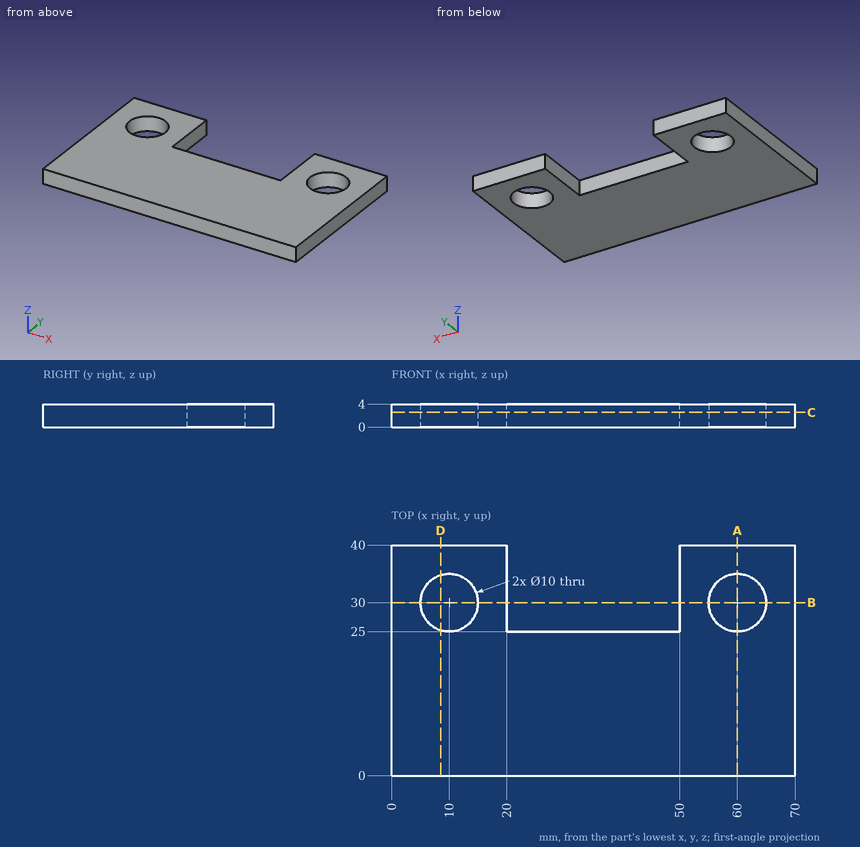
Verification items for this drawing (mm, ordinates from the low corner). Round coordinates to 2 decimals unless told otherwise and drop trailing zeros. Order: outer loops, then holes, each group sorted by start corner. A loop starts at its lowest first (then second) coordinate and runs counter-clockwise, first axis right, second up. Notation, with made-up numbers: M -37.75,31 L -7.75,31 A20 cw -7.75,43 Z; hole C 0.5,28 d11. An arc over 180 degrees is marked long. Answer in a Markdown table with one row per item. Add a question column.
Item 1: Depth check by flat-ended pin: pin 1 Ø1.2 at (x, z) = (31.5, 1.5) entering from +Y. Enter the tip coordinate at first touch or a pass-through.
Item 2: Sectioned sample at A-A, the plane x = 60. Enter the section's corners in (y, z), plus the area to 3 significant figures.
Item 3: Material ranges on L1, parallel to X at y = 30, z = 2.85; L2, parallel to Y at x = 10, z = 1.75; L3, parallel to X at y = 26.5, z = 2.8, recorded low to high. Write a range as [from, to].
Item 4: Sectioned sample at C-C, the plane z = 2.55. Enter the section's corners in (x, y).
Item 5: Sectioned sample at D-D, the plane x = 8.5. Enter the section's corners in (y, z), plus the area to 3 significant figures.
Item 6: Sectioned sample at B-B, the plane y = 30. Enter the section's corners in (x, z), plus the area to 3 significant figures.
Filled in:
| question | item | result |
|---|---|---|
| 1 | pin 1 | stops at y = 25 |
| 2 | outline | M 0,0 L 25,0 L 25,4 L 0,4 Z; M 35,0 L 40,0 L 40,4 L 35,4 Z |
| 2 | area | 120 mm² |
| 3 | L1 | x = [0, 5], [15, 20], [50, 55], [65, 70] |
| 3 | L2 | y = [0, 25], [35, 40] |
| 3 | L3 | x = [0, 6.43], [13.57, 20], [50, 56.43], [63.57, 70] |
| 4 | outline | M 0,0 L 70,0 L 70,40 L 50,40 L 50,25 L 20,25 L 20,40 L 0,40 Z; hole C 10,30 d10; hole C 60,30 d10 |
| 5 | outline | M 0,0 L 25.23,0 L 25.23,4 L 0,4 Z; M 34.77,0 L 40,0 L 40,4 L 34.77,4 Z |
| 5 | area | 122 mm² |
| 6 | outline | M 0,0 L 5,0 L 5,4 L 0,4 Z; M 15,0 L 20,0 L 20,4 L 15,4 Z; M 50,0 L 55,0 L 55,4 L 50,4 Z; M 65,0 L 70,0 L 70,4 L 65,4 Z |
| 6 | area | 80.0 mm² |
